Input: part model. Units: mm. Frame: model coordinates. A direction names the side the tool comes from. Round coordinates to 2 decimals unless told otherwise and drop trailing zeros. Loops run counter-clockwise (first coordinate to the right, second up) from the corner with the lowest first, then second, coordinate; pieces in that order, holes last. Notation, with made-up numbers: M 73,53 L 78,53 A27 ccw 78,70 Z; hole C 64,-2.5 d8. An arc over 180 degrees is marked long. Put each result on its own line as item: value. Start each with the question number.
1) Section B-B on z = 0. Output: boundary loops of the cut face in (x, y) (3 decimals).
2) Section C-C on x = 5.5. Output: boundary loops of the cut face in (y, z), plus the area to 3 significant figures.
3) Draft query along Z for faces 4 (the face through (-2.19, 11.88, -3.73)), 5 (the face through (2, 12, 10)), 6 (the face through (-2.38, 14.71, -10.74)). Return one class per face: +Z half, -Z half, draft (parallel to the pull), parting line (faces both ways), or undercut.
4) Reachability of faces 1 (the face through (5, 17.5, 0)), 2 (the face through (-4.325, 12, 0)), 3 (the face through (0.7, 13, -7.4)) from +Z, -Z, +X, -X, +Y, -Y: full face, straight path, thin tool, end or side. Return the list, or none.
5) Section D-D on z = 8.75. Output: boundary loops of the cut face in (x, y), plus the area to 3 significant figures.
6) Line query: probe 1 along Y at (x, z) = (-7, -6.5); probe 2 along Z at (x, y) = (1, 8.25); probe 3 along Y at (x, z) = (10, -3.75). Output: solid intervals per line, ascending.
7) Pin query (flat end, axial travel): pin 1 (3 mm diameter, centred on y = 10, z = -1.5, fed in from -X) (3 decimals); pin 2 (3 mm diameter, centred on x = 8.5, z = -4.5, fed in from -Y); pin 3 (4 mm diameter, centred on y = 13.5, z = -8.5, fed in from -X). Return the tip coordinate at first contact, or that it passes through.
8) Section A-A on y = 10.75. Output: boundary loops of the cut face in (x, z) (3 decimals).
Autodesk Inventor part; units mm, degrees
ref_plane "YZ Plane" through (0, 0, 0) normal (1, 0, 0) x (0, 1, 0)
ref_plane "XZ Plane" through (0, 0, 0) normal (0, 1, 0) x (-1, 0, 0)
ref_plane "XY Plane" through (0, 0, 0) normal (0, 0, 1) x (1, 0, 0)
sketch "Boceto1" plane through (0, 0, 0) normal (0, 1, 0) x (-1, 0, 0)
  circle A0 centre (0, 0) radius 7.275
  dimension "d0" = 14.55
extrude "Extrusión1" add sketch "Boceto1" along normal blind 12
sketch "Boceto2" plane through (0, 12, 0) normal (0, 1, 0) x (1, 0, 0)
  circle A0 centre (0, 0) radius 11
  dimension "d3" = 22
extrude "Extrusión2" add sketch "Boceto2" along normal blind 5.5
sketch "Boceto3" plane through (0, 17.5, 0) normal (0, 1, 0) x (1, 0, 0)
  line L0 (0, 0) -> (-4.325, 0)
  line L1 (-4.325, 2.497) -> (0, 4.9941)
  line L2 (0, 4.9941) -> (4.325, 2.497)
  line L3 (4.325, 2.497) -> (4.325, -2.497)
  line L4 (4.325, -2.497) -> (0, -4.9941)
  line L5 (0, -4.9941) -> (-4.325, -2.497)
  line L6 (-4.325, -2.497) -> (-4.325, 2.497)
  dimension "d6" = 4.325
extrude "Extrusión3" cut sketch "Boceto3" against normal blind 11.4
thread "Rosca1"
sketch "Boceto4" plane through (0, 12, 0) normal (0, -1, 0) x (1, 0, 0)
  circle A0 centre (0, 0) radius 7.275
  circle A1 centre (0, 0) radius 10
  dimension "d11" = 20
extrude "Extrusión4" cut sketch "Boceto4" against normal blind 1
properties part number "Tuerca_pieza_conectores"
Geometry results:
1. outline: M -11,12 L -10,12 L -10,13 L -7.275,13 L -7.275,0 L 7.275,0 L 7.275,13 L 10,13 L 10,12 L 11,12 L 11,17.5 L 4.325,17.5 L 4.325,6.1 L -4.325,6.1 L -4.325,17.5 L -11,17.5 Z
2. outline: M 0,-4.76 L 13,-4.76 L 13,-8.35 L 12,-8.35 L 12,-9.53 L 17.5,-9.53 L 17.5,9.53 L 12,9.53 L 12,8.35 L 13,8.35 L 13,4.76 L 0,4.76 Z
2. area: 212 mm²
3. face 4: undercut
3. face 5: draft
3. face 6: parting line
4. face 1: +Z, -Z, +X, -X, +Y
4. face 2: +Y
4. face 3: -Y
5. outline: M -6.67,12 L -4.84,12 L -4.84,13 L 4.84,13 L 4.84,12 L 6.67,12 L 6.67,17.5 L -6.67,17.5 Z
5. area: 63.6 mm²
6. probe 1: y = 13 to 17.5
6. probe 2: z = -7.21 to -4.42, 4.42 to 7.21
6. probe 3: y = 12 to 17.5
7. pin 1: stops at x = -7.275
7. pin 2: stops at y = 12
7. pin 3: stops at x = -8.87
8. outline: C 0,0 d14.55; hole M -4.325,-2.497 L 0,-4.994 L 4.325,-2.497 L 4.325,2.497 L 0,4.994 L -4.325,2.497 Z
